Geometry: final body of the model. Coordinates: model frame, mm. Give positions to 0.01 mm unless a question says otherwise; leave off trailing zeros. Write each loop counter-clockwise with the first axis right and the second up, starting at its lowest first coordinate (ties: lowest second). Pieces come first, ordered by that corner, then holes.
Q1. Section A-A (z = 0). Return the cut outline in (x, y).
Q2. Line query: line 1 (X direction, y = -2, z = 0); line 2 (Z direction, x = -15, y = 4.25). Output: solid intervals per line, ascending.
Q3. Section C-C (y = 3). Return the cut outline in (x, z), plus the area to 3 significant figures.
Q4. Section B-B (x = -15). Return the cut outline in (y, z), plus the area to 3 significant figures.
Q5. Mould query, pull axis X, two halves, no side actions, for faces 1 (the cylindrical face through (17.727, 0.14, -0.358)), 2 (the flat face through (-30, 0, 0)), 3 (the flat face through (0, -10, 0)). Classes: +X half, -X half, draft (parallel to the pull), parting line (faces both ways), or undercut.
from build123d import *

# Parameters (mm, degrees)
SKETCH1_W           = 20
SKETCH1_H           = 20
BOSS_EXTRUDE1_DEPTH = 30
SKETCH2_R           = 2.75
CUT_EXTRUDE1_DEPTH  = 38.416573868


with BuildPart() as part:
    # Sketch1 → Boss-Extrude1 (new, symmetric)
    with BuildSketch(Plane(origin=(0, 0, 0), x_dir=(0, 0, -1), z_dir=(1, 0, 0))):
        Rectangle(SKETCH1_W, SKETCH1_H)
    extrude(amount=BOSS_EXTRUDE1_DEPTH, both=True)

    # Sketch2 → Cut-Extrude1 (cut, through all)
    with BuildSketch(Plane(origin=(0, 10, 0), x_dir=(1, 0, 0), z_dir=(0, 1, 0))):
        with Locations(Location((15, 0, 0), (0, 0, 270))):
            Circle(SKETCH2_R)
    cut_extrude1 = extrude(amount=-CUT_EXTRUDE1_DEPTH, mode=Mode.SUBTRACT)

    # Mirror1: Cut-Extrude1 across plane
    add(cut_extrude1.mirror(Plane(origin=(0, 0, 0), x_dir=(0, 0, 1), z_dir=(1, 0, 0))), mode=Mode.SUBTRACT)


solid = part.part
Computed:
1. outline: (-30, -10) - (-17.75, -10) - (-17.75, 10) - (-30, 10) - close; (-12.25, -10) - (12.25, -10) - (12.25, 10) - (-12.25, 10) - close; (17.75, -10) - (30, -10) - (30, 10) - (17.75, 10) - close
2. line 1: x = -30 to -17.75, -12.25 to 12.25, 17.75 to 30
2. line 2: z = -10 to -2.75, 2.75 to 10
3. outline: (-30, -10) - (30, -10) - (30, 10) - (-30, 10) - close; hole circle Ø5.5 at (-15, 0); hole circle Ø5.5 at (15, 0)
3. area: 1,150 mm2
4. outline: (-10, -10) - (10, -10) - (10, -2.75) - (-10, -2.75) - close; (-10, 2.75) - (10, 2.75) - (10, 10) - (-10, 10) - close
4. area: 290 mm2
5. face 1: undercut
5. face 2: -X half
5. face 3: draft
